For this review, take the finished solid that the model builds, in its own axes (mm). Face numbers are marked on the shaded views. A direction names the side the tool comes from. Give positions to 0.01 mm unless a question says otherwise; leave off trailing zeros. Order: outer loops, then holes, each group sorted by start corner. A loop starts at its lowest first (then second) coordinate and runs counter-clockwise, first axis right, second up.
Item 1: For P1, Ø1, axis at x = -6.5, y = -65.5, coming from the +Z side; P2, Ø2, axis at x = -5, y = -72, coming from the -Z side; P3, Ø3, axis at y = -63.5, z = 7.5, coming from the +X side, all flat-tipped, find the tip position at first contact; note any pin that passes through.
Item 2: For probe 1 along Y at (x, z) = (-5, 0); probe 2 along Y at (x, z) = (-8.5, 13); probe 3 along Y at (x, z) = (-6.5, 1.25), list the stretches that pass through material, from the lowest coordinate up.
Item 3: The part is to be moulded in two halves that separate along X. For the marked faces 3, 4, 5 and 6, say which applies: released by +X, released by -X, zero draft, split by the parting line, or undercut.
Item 4: Machinability: for the marked faces 1 and 2, which of the approach directions +Z, -Z, +X, -X, +Y, -Y give a long, thin tool a straight path to every point of the face, cutting with its end or side? Answer none if there is none.
Item 5: Consider section A-A (z = 11). Give the boundary of the cut face in (x, y).
Item 6: Consider section C-C (z = 14.1). Give the boundary of the cut face in (x, y).
Item 7: Consider section B-B (y = -76.5). Give the boundary of the cut face in (x, z).
Item 8: Consider section D-D (x = -1.75). Give the boundary of the cut face in (y, z), plus the area to 3 significant figures.
```python
from build123d import *

# Parameters (mm, degrees)
SKETCH1_W           = 34.2
SKETCH1_H           = 10
SKETCH1_R           = 2.1
BOSS_EXTRUDE1_DEPTH = 3
SKETCH2_W           = 10
SKETCH2_H           = 6
SKETCH2_R           = 2.1
BOSS_EXTRUDE2_DEPTH = 3
SKETCH4_W           = 10
SKETCH4_H           = 6
BOSS_EXTRUDE3_DEPTH = 12
SKETCH5_R           = 2.6
CUT_EXTRUDE1_DEPTH  = 45
SKETCH6_W           = 10
SKETCH6_H           = 22.2
BOSS_EXTRUDE4_DEPTH = 2
BOSS_EXTRUDE5_START = 4
SKETCH7_W           = 10
SKETCH7_H           = 18
SKETCH7_R           = 2.6
BOSS_EXTRUDE5_DEPTH = 4
SKETCH8_W           = 10
SKETCH8_H           = 18
SKETCH8_R           = 2.6
BOSS_EXTRUDE6_DEPTH = 4
BOSS_EXTRUDE7_START = 2
SKETCH10_W          = 10
SKETCH10_H          = 42.2
SKETCH10_R          = 2.1
BOSS_EXTRUDE7_DEPTH = 2


with BuildPart() as part:
    # Sketch1 → Boss-Extrude1 (new body)
    with BuildSketch(Plane(origin=(0, 0, 0), x_dir=(0, 1, 0), z_dir=(0, 0, 1))):
        with Locations((-58.633609256, 5)):
            Rectangle(SKETCH1_W, SKETCH1_H)
        with Locations(Location((-72.733609256, 5, 0), (0, 0, 90))):
            Circle(SKETCH1_R, mode=Mode.SUBTRACT)
        with Locations(Location((-44.533609256, 5, 0), (0, 0, 90))):
            Circle(SKETCH1_R, mode=Mode.SUBTRACT)
    extrude(amount=BOSS_EXTRUDE1_DEPTH)

    # Sketch2 → Boss-Extrude2 (add)
    # profile 1 of 2: a face of its own
    with BuildSketch(Plane.XY.offset(3)):
        with Locations((-5, -44.533609256)):
            Rectangle(SKETCH2_W, SKETCH2_H)
        with Locations(Location((-5, -44.533609256, 0), (0, 0, 180))):
            Circle(SKETCH2_R, mode=Mode.SUBTRACT)
    # profile 2 of 2: a face of its own
    with BuildSketch(Plane.XY.offset(3)):
        with Locations((-5, -72.733609256)):
            Rectangle(SKETCH2_W, SKETCH2_H)
        with Locations(Location((-5, -72.733609256, 0), (0, 0, 180))):
            Circle(SKETCH2_R, mode=Mode.SUBTRACT)
    extrude(amount=BOSS_EXTRUDE2_DEPTH)

    # Sketch4 → Boss-Extrude3 (add)
    with BuildSketch(Plane.XY.offset(6)):
        with Locations((-5, -44.533609256)):
            Rectangle(SKETCH4_W, SKETCH4_H)
        with Locations((-5, -72.733609256)):
            Rectangle(SKETCH4_W, SKETCH4_H)
    extrude(amount=BOSS_EXTRUDE3_DEPTH)

    # Sketch5 → Cut-Extrude1 (cut)
    with BuildSketch(Plane.XZ.offset(75.733609256)):
        with Locations(Location((-5, 14.1, 0), (0, 0, 90))):
            Circle(SKETCH5_R)
    extrude(amount=-CUT_EXTRUDE1_DEPTH, mode=Mode.SUBTRACT)

    # Sketch6 → Boss-Extrude4 (add)
    with BuildSketch(Plane.XY.offset(3)):
        with Locations((-5, -58.633609256)):
            Rectangle(SKETCH6_W, SKETCH6_H)
    extrude(amount=BOSS_EXTRUDE4_DEPTH)

    # Sketch7 → Boss-Extrude5 (add)
    with BuildSketch(Plane.XZ.offset(75.733609256).offset(BOSS_EXTRUDE5_START)):
        with Locations((-5, 9)):
            Rectangle(SKETCH7_W, SKETCH7_H)
        with Locations(Location((-5, 14.1, 0), (0, 0, 90))):
            Circle(SKETCH7_R, mode=Mode.SUBTRACT)
    extrude(amount=-BOSS_EXTRUDE5_DEPTH)

    # Sketch8 → Boss-Extrude6 (add)
    with BuildSketch(Plane(origin=(0, -41.533609256, 0), x_dir=(-1, 0, 0), z_dir=(0, 1, 0))):
        with Locations((5, 9)):
            Rectangle(SKETCH8_W, SKETCH8_H)
        with Locations(Location((5, 14.1, 0), (0, 0, 90))):
            Circle(SKETCH8_R, mode=Mode.SUBTRACT)
    extrude(amount=BOSS_EXTRUDE6_DEPTH)

    # Sketch10 → Boss-Extrude7 (add)
    with BuildSketch(Plane(origin=(0, 0, 0), x_dir=(1, 0, 0), z_dir=(0, 0, -1)).offset(BOSS_EXTRUDE7_START)):
        with Locations((-5, 58.633609256)):
            Rectangle(SKETCH10_W, SKETCH10_H)
        with Locations(Location((-5, 72.733609256, 0), (0, 0, 180))):
            Circle(SKETCH10_R, mode=Mode.SUBTRACT)
        with Locations(Location((-5, 44.533609256, 0), (0, 0, 180))):
            Circle(SKETCH10_R, mode=Mode.SUBTRACT)
    extrude(amount=-BOSS_EXTRUDE7_DEPTH)


solid = part.part
```
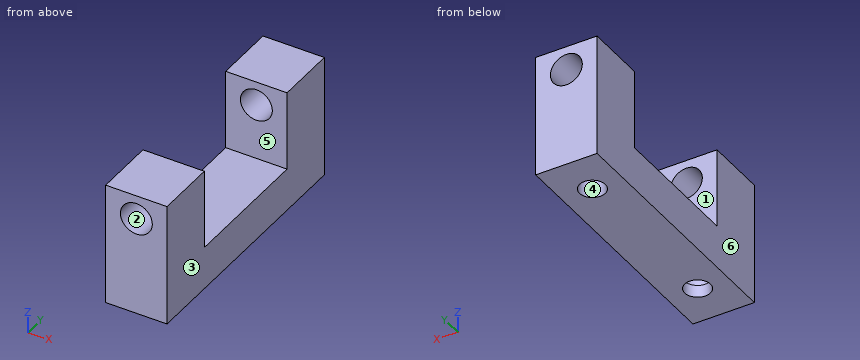
Resolved:
1. P1: stops at z = 5
1. P2: stops at z = 6
1. P3: passes through
2. probe 1: y = -79.73 to -74.83, -70.63 to -46.63, -42.43 to -37.53
2. probe 2: y = -79.73 to -69.73, -47.53 to -37.53
2. probe 3: y = -79.73 to -74.2, -71.26 to -46, -43.06 to -37.53
3. face 3: released by +X
3. face 4: undercut
3. face 5: zero draft
3. face 6: released by -X
4. face 1: +Z, +X, -X
4. face 2: +Y, -Y
5. outline: (-10, -79.73) - (0, -79.73) - (0, -69.73) - (-10, -69.73) - close; (-10, -47.53) - (0, -47.53) - (0, -37.53) - (-10, -37.53) - close
6. outline: (-10, -79.73) - (-7.6, -79.73) - (-7.6, -69.73) - (-10, -69.73) - close; (-10, -47.53) - (-7.6, -47.53) - (-7.6, -37.53) - (-10, -37.53) - close; (-2.4, -79.73) - (0, -79.73) - (0, -69.73) - (-2.4, -69.73) - close; (-2.4, -47.53) - (0, -47.53) - (0, -37.53) - (-2.4, -37.53) - close
7. outline: (-10, -2) - (0, -2) - (0, 18) - (-10, 18) - close; hole circle Ø5.2 at (-5, 14.1)
8. outline: (-79.73, -2) - (-37.53, -2) - (-37.53, 18) - (-47.53, 18) - (-47.53, 5) - (-69.73, 5) - (-69.73, 18) - (-79.73, 18) - close
8. area: 555 mm2
